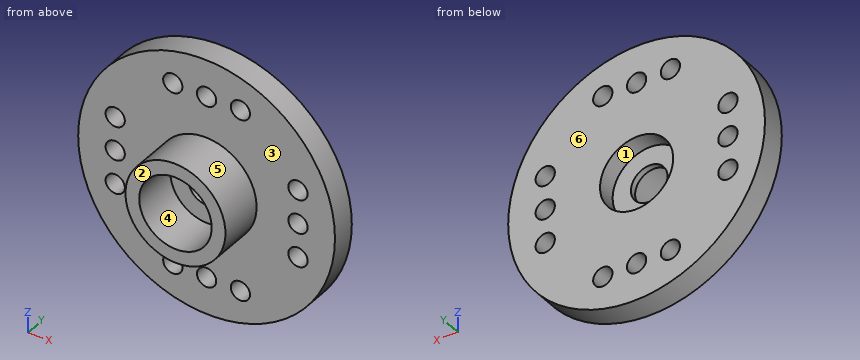
from build123d import *

# Parameters (mm, degrees)
SKETCH_1_R           = 10.525
EXTRUDE_1_DEPTH      = 2
SKETCH_2_R           = 4.1
EXTRUDE_2_DEPTH      = 3.7
SKETCH_3_R           = 2.97
CUT_EXTRUDE_1_DEPTH  = 3.7
SKETCH_4_R           = 1.5
CUT_EXTRUDE_2_DEPTH  = 2
SKETCH_5_R           = 3
CUT_EXTRUDE_3_DEPTH  = 1.5
SKETCH_6_R           = 0.79
CUT_EXTRUDE_4_DEPTH  = 2
SKETCH_7_R           = 0.79
CUT_EXTRUDE_5_DEPTH  = 2
SKETCH_8_R           = 0.79
CUT_EXTRUDE_6_DEPTH  = 2
SKETCH_9_R           = 0.79
CUT_EXTRUDE_7_DEPTH  = 2
SKETCH_10_R          = 0.79
CUT_EXTRUDE_8_DEPTH  = 2
SKETCH_11_R          = 0.79
CUT_EXTRUDE_9_DEPTH  = 2
SKETCH_12_R          = 0.79
CUT_EXTRUDE_10_DEPTH = 2
SKETCH_13_R          = 0.79
CUT_EXTRUDE_11_DEPTH = 2
SKETCH_14_R          = 0.79
CUT_EXTRUDE_12_DEPTH = 2
SKETCH_15_R          = 0.79
CUT_EXTRUDE_13_DEPTH = 2
SKETCH_16_R          = 0.79
CUT_EXTRUDE_14_DEPTH = 2
SKETCH_17_R          = 0.79
CUT_EXTRUDE_15_DEPTH = 2


with BuildPart() as part:
    # ｽｹｯﾁ1 → ﾎﾞｽ - 押し出し1 (new body)
    with BuildSketch(Plane(origin=(0, 0, 0), x_dir=(1, 0, 0), z_dir=(0, 1, 0))):
        Circle(SKETCH_1_R)
    extrude(amount=EXTRUDE_1_DEPTH)

    # ｽｹｯﾁ2 → ﾎﾞｽ - 押し出し2 (add)
    with BuildSketch(Plane(origin=(0, 0, 0), x_dir=(-1, 0, 0), z_dir=(0, -1, 0))):
        Circle(SKETCH_2_R)
    extrude(amount=EXTRUDE_2_DEPTH)

    # ｽｹｯﾁ3 → ｶｯﾄ - 押し出し1 (cut)
    with BuildSketch(Plane(origin=(0, -3.7, 0), x_dir=(-1, 0, 0), z_dir=(0, -1, 0))):
        Circle(SKETCH_3_R)
    extrude(amount=-CUT_EXTRUDE_1_DEPTH, mode=Mode.SUBTRACT)

    # ｽｹｯﾁ4 → ｶｯﾄ - 押し出し2 (cut)
    with BuildSketch(Plane(origin=(0, 2, 0), x_dir=(1, 0, 0), z_dir=(0, 1, 0))):
        Circle(SKETCH_4_R)
    extrude(amount=-CUT_EXTRUDE_2_DEPTH, mode=Mode.SUBTRACT)

    # ｽｹｯﾁ5 → ｶｯﾄ - 押し出し3 (cut)
    with BuildSketch(Plane(origin=(0, 2, 0), x_dir=(1, 0, 0), z_dir=(0, 1, 0))):
        Circle(SKETCH_5_R)
    extrude(amount=-CUT_EXTRUDE_3_DEPTH, mode=Mode.SUBTRACT)

    # ｽｹｯﾁ6 → ｶｯﾄ - 押し出し4 (cut)
    with BuildSketch(Plane(origin=(0, 2, 0), x_dir=(1, 0, 0), z_dir=(0, 1, 0))):
        with Locations((0, 7.49)):
            Circle(SKETCH_6_R)
    extrude(amount=-CUT_EXTRUDE_4_DEPTH, mode=Mode.SUBTRACT)

    # ｽｹｯﾁ7 → ｶｯﾄ - 押し出し5 (cut)
    with BuildSketch(Plane(origin=(0, 2, 0), x_dir=(1, 0, 0), z_dir=(0, 1, 0))):
        with Locations((2.77, 7.49)):
            Circle(SKETCH_7_R)
    extrude(amount=-CUT_EXTRUDE_5_DEPTH, mode=Mode.SUBTRACT)

    # ｽｹｯﾁ8 → ｶｯﾄ - 押し出し6 (cut)
    with BuildSketch(Plane(origin=(0, 2, 0), x_dir=(1, 0, 0), z_dir=(0, 1, 0))):
        with Locations((-2.77, 7.49)):
            Circle(SKETCH_8_R)
    extrude(amount=-CUT_EXTRUDE_6_DEPTH, mode=Mode.SUBTRACT)

    # ｽｹｯﾁ9 → ｶｯﾄ - 押し出し7 (cut)
    with BuildSketch(Plane(origin=(0, 2, 0), x_dir=(1, 0, 0), z_dir=(0, 1, 0))):
        with Locations((7.49, 0)):
            Circle(SKETCH_9_R)
    extrude(amount=-CUT_EXTRUDE_7_DEPTH, mode=Mode.SUBTRACT)

    # ｽｹｯﾁ10 → ｶｯﾄ - 押し出し8 (cut)
    with BuildSketch(Plane(origin=(0, 2, 0), x_dir=(1, 0, 0), z_dir=(0, 1, 0))):
        with Locations((7.49, -2.77)):
            Circle(SKETCH_10_R)
    extrude(amount=-CUT_EXTRUDE_8_DEPTH, mode=Mode.SUBTRACT)

    # ｽｹｯﾁ11 → ｶｯﾄ - 押し出し9 (cut)
    with BuildSketch(Plane(origin=(0, 2, 0), x_dir=(1, 0, 0), z_dir=(0, 1, 0))):
        with Locations((7.49, 2.77)):
            Circle(SKETCH_11_R)
    extrude(amount=-CUT_EXTRUDE_9_DEPTH, mode=Mode.SUBTRACT)

    # ｽｹｯﾁ12 → ｶｯﾄ - 押し出し10 (cut)
    with BuildSketch(Plane(origin=(0, 2, 0), x_dir=(1, 0, 0), z_dir=(0, 1, 0))):
        with Locations((0, -7.49)):
            Circle(SKETCH_12_R)
    extrude(amount=-CUT_EXTRUDE_10_DEPTH, mode=Mode.SUBTRACT)

    # ｽｹｯﾁ13 → ｶｯﾄ - 押し出し11 (cut)
    with BuildSketch(Plane(origin=(0, 2, 0), x_dir=(1, 0, 0), z_dir=(0, 1, 0))):
        with Locations((2.77, -7.49)):
            Circle(SKETCH_13_R)
    extrude(amount=-CUT_EXTRUDE_11_DEPTH, mode=Mode.SUBTRACT)

    # ｽｹｯﾁ14 → ｶｯﾄ - 押し出し12 (cut)
    with BuildSketch(Plane(origin=(0, 2, 0), x_dir=(1, 0, 0), z_dir=(0, 1, 0))):
        with Locations((-2.77, -7.49)):
            Circle(SKETCH_14_R)
    extrude(amount=-CUT_EXTRUDE_12_DEPTH, mode=Mode.SUBTRACT)

    # ｽｹｯﾁ15 → ｶｯﾄ - 押し出し13 (cut)
    with BuildSketch(Plane(origin=(0, 2, 0), x_dir=(1, 0, 0), z_dir=(0, 1, 0))):
        with Locations((-7.49, 0)):
            Circle(SKETCH_15_R)
    extrude(amount=-CUT_EXTRUDE_13_DEPTH, mode=Mode.SUBTRACT)

    # ｽｹｯﾁ16 → ｶｯﾄ - 押し出し14 (cut)
    with BuildSketch(Plane(origin=(0, 2, 0), x_dir=(1, 0, 0), z_dir=(0, 1, 0))):
        with Locations((-7.49, 2.77)):
            Circle(SKETCH_16_R)
    extrude(amount=-CUT_EXTRUDE_14_DEPTH, mode=Mode.SUBTRACT)

    # ｽｹｯﾁ17 → ｶｯﾄ - 押し出し15 (cut)
    with BuildSketch(Plane(origin=(0, 2, 0), x_dir=(1, 0, 0), z_dir=(0, 1, 0))):
        with Locations((-7.49, -2.77)):
            Circle(SKETCH_17_R)
    extrude(amount=-CUT_EXTRUDE_15_DEPTH, mode=Mode.SUBTRACT)


solid = part.part
Model file for the job. Use its own axes, mm. Face numbers are marked on the shaded views. A direction names the side the tool comes from. Give positions to 0.01 mm unless a question says otherwise; leave off trailing zeros. Write each loop counter-clockwise with the first axis right and the second up, starting at its lowest first coordinate (ties: lowest second). Pieces come first, ordered by that corner, then holes. Notation, with made-up numbers: (-40, 80) - (8, 80) arc R28 cw to (8, 104) - close; hole circle Ø5 at (-23.5, 22.25). An arc over 180 degrees is marked (long way). Answer as CSV lines item,"result".
1. Band-saw the part on A-A (x = 0). Write the cut outline in (y, z) (3 decimals).
Responses:
outline,"(-3.7, -4.1) - (0, -4.1) - (0, -6.7) - (2, -6.7) - (2, -3) - (0.5, -3) - (0.5, -1.5) - (0, -1.5) - (0, -2.97) - (-3.7, -2.97) - close; (-3.7, 2.97) - (0, 2.97) - (0, 1.5) - (0.5, 1.5) - (0.5, 3) - (2, 3) - (2, 6.7) - (0, 6.7) - (0, 4.1) - (-3.7, 4.1) - close; (0, -10.525) - (2, -10.525) - (2, -8.28) - (0, -8.28) - close; (0, 8.28) - (2, 8.28) - (2, 10.525) - (0, 10.525) - close"
2. Pin check, flat tips, straight feed: pin 1 (0.9 mm diameter, centred on x = -7.49, z = 2.77, fed in from +Y); pin 2 (5 mm diameter, centred on x = 0, z = 0, fed in from -Y). Stop position of each tip, or through.
Responses:
pin 1,"passes through"
pin 2,"stops at y = 0"
3. 3-axis set-ups, long thin cutter, end or side, ignore diameter. For the marked faces 1, 2 and 3: which of +Z, -Z, +X, -X, +Y, -Y reach the whole face in a straight line?
Responses:
face 1,"+Y"
face 2,"+Z, -Z, +X, -X, -Y"
face 3,"-Y"
4. Band-saw the part on B-B (y = 0.95). Count the separate pieces of the cut face and the enclosed holes in it, and give its area (3 significant figures).
Responses:
separate pieces,"1"
enclosed holes,"13"
area,"296 mm2"
5. Band-saw the part on D-D (y = -1.85). Write the cut outline in (x, z).
Responses:
outline,"circle Ø8.2 at (0, 0); hole circle Ø5.94 at (0, 0)"
6. Drill centre lines: L1, parallel to Z at x = 0, y = 1 (3 decimals); L2, parallel to X at y = -2.7, z = 0. Where is each one in solid material? Low to high. Write a range as [from, to].
Responses:
L1,"z = [-10.525, -8.28], [-6.7, -3], [3, 6.7], [8.28, 10.525]"
L2,"x = [-4.1, -2.97], [2.97, 4.1]"
7. Band-saw the part on C-C (z = 7.49). Write the cut outline in (x, y).
Responses:
outline,"(-7.39, 0) - (-3.56, 0) - (-3.56, 2) - (-7.39, 2) - close; (-1.98, 0) - (-0.79, 0) - (-0.79, 2) - (-1.98, 2) - close; (0.79, 0) - (1.98, 0) - (1.98, 2) - (0.79, 2) - close; (3.56, 0) - (7.39, 0) - (7.39, 2) - (3.56, 2) - close"
8. Two-plate mould, pull along Z, no slides. Class the marked faces 4, 5 and 6: +Z half, -Z half, draft (parallel to the pull), parting line (faces both ways), or undercut.
Responses:
face 4,"undercut"
face 5,"parting line"
face 6,"draft"
